Geometry check sheet. Reference: the model listing, model coordinates, mm. A direction names the side the tool comes from. Give positions to 0.01 mm unless a question says otherwise; leave off trailing zeros. Order: outer loops, then holes, each group sorted by start corner. A loop starts at its lowest first (then second) coordinate and runs counter-clockwise, first axis right, second up. Notation, with made-up numbers: M -23,63.5 L 8,63.5 A31 cw 8,95.5 Z; hole C -34,53.5 d7. An arc over 180 degrees is marked long. Answer as CSV lines item,"result". Start each with the question number.
Q1. Thickness scan on line 1 (X direction, y = 30.5, z = -103); line 2 (X direction, y = 15.5, z = -153.5); line 3 (Y direction, x = 33.5, z = -55). Record the ranges inside material, lowest first.
Q2. Go/stop test with flat-tipped pins: pin 1 (1.5 mm diameter, centred on x = 4, z = -182.5, fed in from +Y); pin 2 (8 mm diameter, centred on x = 10, z = -96, fed in from +Y); pin 3 (0.5 mm diameter, centred on y = 30, z = -142, fed in from +X). Record where each tip stops, or that it passes through.
Q3. Mould release check, pull along X, two halves, no side actions. Record for faces 4 (the flat face through (20, 1.5, -99)), 5 (the cylindrical face through (1.141, 1.203, -98.813)), 6 (the flat face through (34.5, 34, -99)), 7 (the flat face through (20, 0, -99)): +X half, -X half, draft (parallel to the pull), parting line (faces both ways), or undercut.
Q4. Set-up check for faces 1 (the flat face through (0, 16, -99)), 2 (the flat face through (38.5, 17, -99)), 3 (the flat face through (5.5, 34, -99)): record each of +Z, -Z, +X, -X, +Y, -Y from which the full face is reachable in a straight line by a thin tool's end or side.
Q5. Section check A-A, the plane y = 14.5. Record the boundary of the cut face in (x, z).
Q6. Section check B-B, the plane x = 25. Record the boundary of the cut face in (y, z), then the cut area to 4 significant figures.
```python
from build123d import *

# Parameters (mm, degrees)
BOSS_EXTRUDE1_DEPTH = 241


with BuildPart() as part:
    # Sketch1 → Boss-Extrude1 (new body)
    with BuildSketch(Plane.XY.offset(20)):
        with BuildLine():
            Line((4, 0), (36, 0))
            ThreePointArc((36, 0), (38.828427125, 1.171572875), (40, 4))
            Line((40, 4), (40, 27.499999994))
            ThreePointArc((40, 27.499999994), (39.56066017, 28.56066017), (38.499999994, 29))
            Line((38.499999994, 29), (37.408493132, 29))
            ThreePointArc((37.408493132, 29), (37.05493974, 29.14644661), (36.90849313, 29.500000002))
            Line((36.90849313, 29.500000002), (36.90849313, 30.572020267))
            ThreePointArc((36.90849313, 30.572020267), (36.86079319, 30.785150869), (36.726794508, 30.957616203))
            ThreePointArc((36.726794508, 30.957616203), (36.005111578, 32.357100716), (36.519951827, 33.845160752))
            ThreePointArc((36.519951827, 33.845160752), (36.647077826, 34.128030253), (36.582952488, 34.431450944))
            Line((36.582952488, 34.431450944), (35.099999998, 37.000000001))
            Line((35.099999998, 37.000000001), (34.500000002, 37.000000001))
            Line((34.500000002, 37.000000001), (34.500000002, 30.672689193))
            Line((34.500000002, 30.672689193), (34.158493132, 30.561067543))
            Line((34.158493132, 30.561067543), (34.158493132, 29.989862813))
            Line((34.158493132, 29.989862813), (34.908493132, 29.989862813))
            Line((34.908493132, 29.989862813), (34.908493132, 29.700000011))
            ThreePointArc((34.908493132, 29.700000011), (35.494279572, 28.285786443), (36.908493141, 27.700000003))
            Line((36.908493141, 27.700000003), (38.000000017, 27.700000003))
            ThreePointArc((38.000000017, 27.700000003), (38.353553409, 27.553553393), (38.500000019, 27.200000001))
            Line((38.500000019, 27.200000001), (38.500000019, 6.9547727))
            ThreePointArc((38.500000019, 6.9547727), (37.882683451, 6.030893167), (36.792893237, 6.247665919))
            Line((36.792893237, 6.247665919), (36.648161659, 6.392397496))
            ThreePointArc((36.648161659, 6.392397496), (35.587251229, 8.859212237), (33.009530056, 9.611581471))
            ThreePointArc((33.009530056, 9.611581471), (32.804700675, 9.478725012), (32.766463725, 9.237594653))
            Line((32.766463725, 9.237594653), (33.047066675, 8.190370192))
            ThreePointArc((33.047066675, 8.190370192), (34.786339421, 7.686520507), (35.148364083, 5.912296075))
            Line((35.148364083, 5.912296075), (36.146446608, 4.91421355))
            ThreePointArc((36.146446608, 4.91421355), (36.292893217, 4.560660161), (36.146446608, 4.207106773))
            Line((36.146446608, 4.207106773), (35.792893214, 3.853553379))
            ThreePointArc((35.792893214, 3.853553379), (35.439339826, 3.70710677), (35.085786437, 3.853553379))
            Line((35.085786437, 3.853553379), (34.087703906, 4.85163591))
            ThreePointArc((34.087703906, 4.85163591), (32.313479487, 5.213660585), (31.809629807, 6.952933321))
            Line((31.809629807, 6.952933321), (30.762405333, 7.233536272))
            ThreePointArc((30.762405333, 7.233536272), (30.521274984, 7.195299323), (30.38841853, 6.990469949))
            ThreePointArc((30.38841853, 6.990469949), (31.140787752, 4.412748784), (33.607602477, 3.351838341))
            Line((33.607602477, 3.351838341), (33.752334032, 3.207106785))
            ThreePointArc((33.752334032, 3.207106785), (33.969106782, 2.117316579), (33.045227255, 1.500000015))
            Line((33.045227255, 1.500000015), (6.954772716, 1.500000015))
            ThreePointArc((6.954772716, 1.500000015), (6.030893183, 2.117316583), (6.247665934, 3.207106797))
            Line((6.247665934, 3.207106797), (6.392397512, 3.351838375))
            ThreePointArc((6.392397512, 3.351838375), (8.859212224, 4.412748803), (9.611581449, 6.990469949))
            ThreePointArc((9.611581449, 6.990469949), (9.478724996, 7.195299323), (9.237594646, 7.233536272))
            Line((9.237594646, 7.233536272), (8.190370187, 6.952933328))
            ThreePointArc((8.190370187, 6.952933328), (7.686520502, 5.213660596), (5.912296085, 4.851635932))
            Line((5.912296085, 4.851635932), (4.914213553, 3.8535534))
            ThreePointArc((4.914213553, 3.8535534), (4.560660164, 3.707106791), (4.207106776, 3.8535534))
            Line((4.207106776, 3.8535534), (3.853553388, 4.207106787))
            ThreePointArc((3.853553388, 4.207106787), (3.70710678, 4.560660175), (3.853553388, 4.914213564))
            Line((3.853553388, 4.914213564), (4.85163592, 5.912296095))
            ThreePointArc((4.85163592, 5.912296095), (5.213660585, 7.686520517), (6.952933322, 8.190370198))
            Line((6.952933322, 8.190370198), (7.233536268, 9.237594644))
            ThreePointArc((7.233536268, 9.237594644), (7.195299318, 9.478725003), (6.990469936, 9.611581462))
            ThreePointArc((6.990469936, 9.611581462), (4.412748785, 8.859212233), (3.351838362, 6.392397513))
            Line((3.351838362, 6.392397513), (3.207106785, 6.247665935))
            ThreePointArc((3.207106785, 6.247665935), (2.11731657, 6.030893183), (1.500000002, 6.954772717))
            Line((1.500000002, 6.954772717), (1.500000002, 27.200000001))
            ThreePointArc((1.500000002, 27.200000001), (1.646446612, 27.553553393), (2.000000004, 27.700000003))
            Line((2.000000004, 27.700000003), (3.091506864, 27.700000003))
            ThreePointArc((3.091506864, 27.700000003), (4.505720432, 28.285786443), (5.091506872, 29.700000011))
            Line((5.091506872, 29.700000011), (5.091506872, 29.989862813))
            Line((5.091506872, 29.989862813), (5.841506868, 29.989862813))
            Line((5.841506868, 29.989862813), (5.841506868, 30.561067541))
            Line((5.841506868, 30.561067541), (5.499999998, 30.672689191))
            Line((5.499999998, 30.672689191), (5.499999998, 37.000000001))
            Line((5.499999998, 37.000000001), (4.899999998, 37.000000001))
            Line((4.899999998, 37.000000001), (3.417047508, 34.431450944))
            ThreePointArc((3.417047508, 34.431450944), (3.35292217, 34.128030253), (3.480048169, 33.845160751))
            ThreePointArc((3.480048169, 33.845160751), (3.99488842, 32.357100716), (3.273205491, 30.957616203))
            ThreePointArc((3.273205491, 30.957616203), (3.13920681, 30.785150869), (3.09150687, 30.572020267))
            Line((3.09150687, 30.572020267), (3.09150687, 29.500000002))
            ThreePointArc((3.09150687, 29.500000002), (2.94506026, 29.14644661), (2.591506868, 29))
            Line((2.591506868, 29), (1.500000006, 29))
            ThreePointArc((1.500000006, 29), (0.43933983, 28.56066017), (0, 27.499999994))
            Line((0, 27.499999994), (0, 4))
            ThreePointArc((0, 4), (1.171572875, 1.171572875), (4, 0))
        make_face()
    extrude(amount=-BOSS_EXTRUDE1_DEPTH)


solid = part.part
```
Answer block:
1,line 1,"x = 3.09 to 5.84, 34.16 to 36.91"
1,line 2,"x = 0 to 1.5, 38.5 to 40"
1,line 3,"y = 0 to 1.61, 3.35 to 4.75, 8.25 to 9.65"
2,pin 1,"stops at y = 36.74"
2,pin 2,"stops at y = 9.65"
2,pin 3,"stops at x = 36.91"
3,face 4,"undercut"
3,face 5,"-X half"
3,face 6,"undercut"
3,face 7,"draft"
4,face 1,"+Z, -Z, -X, +Y, -Y"
4,face 2,"+Z, -Z"
4,face 3,"+Z, -Z, +Y"
5,outline,"M 0,-221 L 1.5,-221 L 1.5,20 L 0,20 Z; M 38.5,-221 L 40,-221 L 40,20 L 38.5,20 Z"
6,outline,"M 0,-221 L 1.5,-221 L 1.5,20 L 0,20 Z"
6,area,"361.5 mm2"
